Geometry check sheet. Reference: drawing and pictorial views, mm from the part's lowest x, y, z. Round coordinates to 2 decimals unless told otherwise and drop trailing zeros. Loops run counter-clockwise (first coordinate to the right, second up) from the corner with the lowest first, then second, coordinate; pieces in that order, holes last. Notation, with made-up numbers: (64, 77.25) - (69, 77.25) arc R24 cw to (69, 95.25) - close; hole circle Ø5 at (18, -34.75). An arc over 180 degrees is marked (long way). Answer as CSV lines item,"result". Start each with the question number.
1) Thickness scan on line 1 along Y through (x, z) = (1.4, 44); line 2 along Z through (x, y) = (2.55, 6.5); line 3 along Y through (x, z) = (2.1, 6). Record the ranges inside material, lowest first.
2) Depth check by flat-ended pin: P1, Ø2, axis at x = 1, y = 10.5, coming from the +Z side. Enter the tip coordinate at first touch or a pass-through.
3) Cross-section at B-B on x = 2.15. Record the boundary of the cut face in (y, z).
4) Cross-section at A-A on z = 44. Record the boundary of the cut face in (x, y).
5) Cross-section at C-C on y = 6. Record the boundary of the cut face in (x, z).
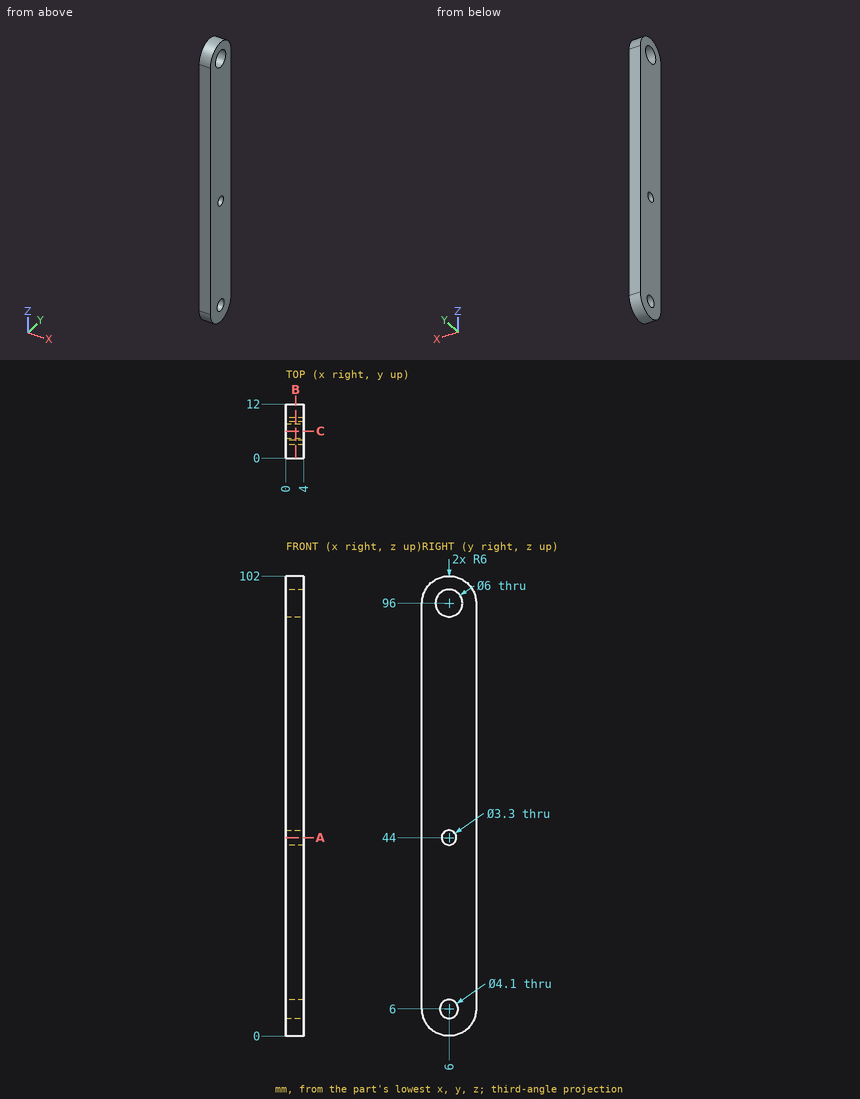
Answer block:
1,line 1,"y = 0 to 4.35, 7.65 to 12"
1,line 2,"z = 0.02 to 4.01, 7.99 to 42.43, 45.57 to 93.04, 98.96 to 101.98"
1,line 3,"y = 0 to 3.95, 8.05 to 12"
2,P1,"stops at z = 100.87"
3,outline,"(0, 6) arc R6 ccw to (12, 6) - (12, 96) arc R6 ccw to (0, 96) - close; hole circle Ø6 at (6, 96); hole circle Ø4.1 at (6, 6); hole circle Ø3.3 at (6, 44)"
4,outline,"(0, 0) - (4, 0) - (4, 4.35) - (0, 4.35) - close; (0, 7.65) - (4, 7.65) - (4, 12) - (0, 12) - close"
5,outline,"(0, 0) - (4, 0) - (4, 3.95) - (0, 3.95) - close; (0, 8.05) - (4, 8.05) - (4, 42.35) - (0, 42.35) - close; (0, 45.65) - (4, 45.65) - (4, 93) - (0, 93) - close; (0, 99) - (4, 99) - (4, 102) - (0, 102) - close"
